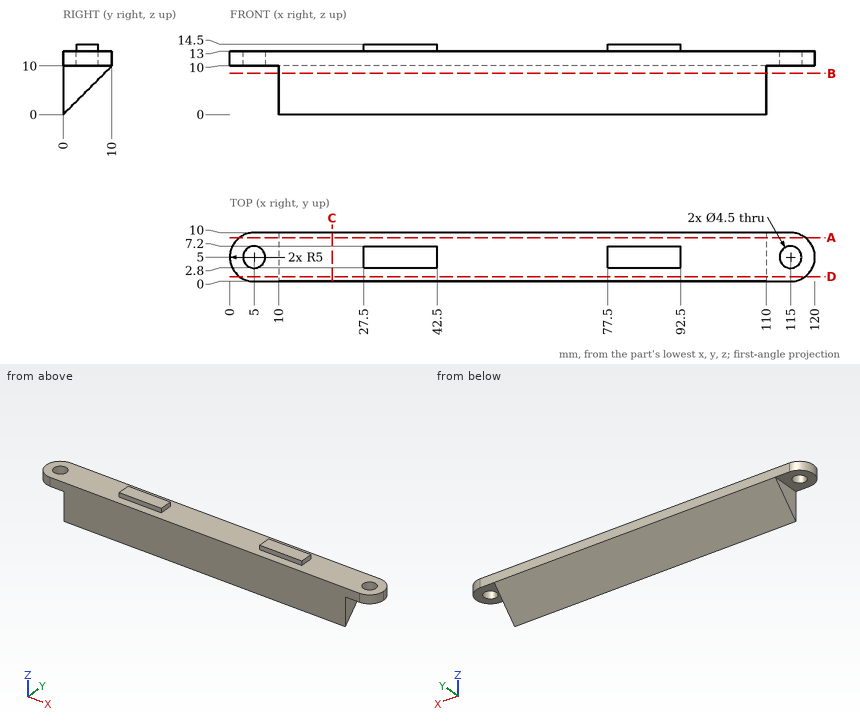
Design review of the part shown in the three views and the two pictorial views. Dimensions are in mm from the part's minimum x, y and z. Round coordinates to 2 decimals unless told otherwise and drop trailing zeros. Write each loop counter-clockwise with the first axis right and the second up, starting at its lowest first coordinate (ties: lowest second). Pieces come first, ordered by that corner, then holes.
1) For line 1 along Y through (x, z) = (5, 11.75); line 2 along Z through (x, y) = (97.5, 5); line 3 along X through (y, z) = (5.5, 6.25), list the stretches that pass through material, from the lowest coordinate up.
Answer below:
line 1: y = 0 to 2.75, 7.25 to 10
line 2: z = 5 to 13
line 3: x = 10 to 110
2) Insertion check: pin 1 Ø5 at (y, z) = (7.5, 9) entering from +X; pin 2 Ø1.2 at (y, z) = (6, 13.5) entering from -X; pin 3 Ø4 at (x, y) = (115, 5) entering from +Z; pin 4 Ø0.8 at (y, z) = (5, 13.5) entering from -X. Each pin has a flat end and moves straight along its axis. Give the tip position at first contact, or say it passes through.
Answer below:
pin 1: stops at x = 120
pin 2: stops at x = 0.04
pin 3: passes through
pin 4: stops at x = 27.5
3) Take a section at D-D on y = 1. Give the boundary of the cut face in (x, z).
Answer below:
outline: (2, 10) - (10, 10) - (10, 1) - (110, 1) - (110, 10) - (118, 10) - (118, 13) - (2, 13) - close
4) Take a section at C-C on x = 21. Give the boundary of the cut face in (y, z).
Answer below:
outline: (0, 0) - (10, 10) - (10, 13) - (0, 13) - close
5) Take a section at A-A on y = 9. Give the boundary of the cut face in (x, z), then the cut area to 3 significant figures.
Answer below:
outline: (2, 10) - (10, 10) - (10, 9) - (110, 9) - (110, 10) - (118, 10) - (118, 13) - (2, 13) - close
area: 448 mm2
6) Take a section at B-B on z = 8.5. Give the boundary of the cut face in (x, y).
Answer below:
outline: (10, 0) - (110, 0) - (110, 8.5) - (10, 8.5) - close
